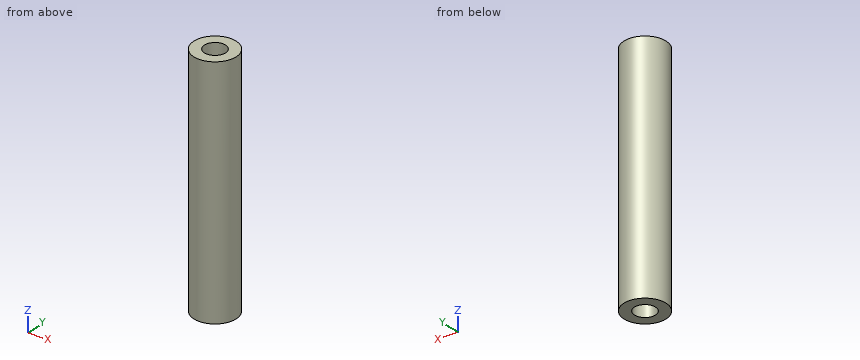
Autodesk Inventor part; units mm, degrees
ref_plane "YZ Plane" through (0, 0, 0) normal (1, 0, 0) x (0, 1, 0)
ref_plane "XZ Plane" through (0, 0, 0) normal (0, 1, 0) x (-1, 0, 0)
ref_plane "XY Plane" through (0, 0, 0) normal (0, 0, 1) x (1, 0, 0)
sketch "スケッチ1" plane through (0, 0, 0) normal (0, 0, 1) x (1, 0, 0)
  circle A0 centre (0, 0) radius 4
  dimension "d0" = 8
extrude "押し出し1" add sketch "スケッチ1" along normal blind 45
hole "穴1" at (0, 0, 0) direction (0, 0, 1) diameter 4 depth 8 tip angle 118
sketch "スケッチ2" plane through (0, 0, 45) normal (0, 0, 1) x (1, 0, 0)
  point P0 (0, 0)
  point P1 (0, 0)
hole "穴2" at (0, 0, 45) direction (0, 0, -1) diameter 4 depth 8 tip angle 118
properties part number "スペーサ　m4-l45" material "アルミニウム 2014-T4"
Work out the finished part from the listing and answer in its coordinate system (mm). Coordinates: 2 decimals unless noted, no trailing zeros. Order: outer loops, then holes, each group sorted by start corner. A loop starts at its lowest first (then second) coordinate and runs counter-clockwise, first axis right, second up. Notation, with made-up numbers: (-31.5, 46) - (23.5, 46) arc R14 ccw to (23.5, 65) - close; hole circle Ø2 at (-3.5, -2.75). An arc over 180 degrees is marked (long way). Answer as a JSON object with one key per item and string values.
1. Consider line 1 (Y direction, x = 0, z = 39.5); line 2 (X direction, y = 1.25, z = 38); line 3 (X direction, y = -1.5, z = 5). Determine where each line is inside the solid, lowest interval first.
Output values:
{"line 1": "y = -4 to -2, 2 to 4", "line 2": "x = -3.8 to -1.56, 1.56 to 3.8", "line 3": "x = -3.71 to -1.32, 1.32 to 3.71"}
2. Each of these flat-tipped pins is pushed along its axis until it touches: P1, Ø4, axis at x = 2, y = -0.5, coming from the -Z side; P2, Ø3, axis at x = 0, y = 0, coming from the +Z side; P3, Ø3.5, axis at x = 0, y = 0, coming from the +Z side. Where does it stop, or does it pass through?
Output values:
{"P1": "stops at z = 0", "P2": "stops at z = 36.7", "P3": "stops at z = 36.85"}
3. Find section C-C on z = 26. Determine the outline of the cut face in (x, y).
Output values:
{"outline": "circle Ø8 at (0, 0)"}
4. Find section D-D on y = -2.5. Determine the outline of the cut face in (x, z), plus the area to 3 significant figures.
Output values:
{"outline": "(-3.12, 0) - (3.12, 0) - (3.12, 45) - (-3.12, 45) - close", "area": "281 mm²"}
5. Find section A-A on z = 6.5. Determine the outline of the cut face in (x, y).
Output values:
{"outline": "circle Ø8 at (0, 0); hole circle Ø4 at (0, 0)"}
6. Find section B-B on x = 3. Determine the outline of the cut face in (y, z), plus the area to 3 significant figures.
Output values:
{"outline": "(-2.65, 0) - (2.65, 0) - (2.65, 45) - (-2.65, 45) - close", "area": "238 mm²"}
